Here's how the part is built. I have some questions about the finished solid (model axes, mm). Face numbers are marked on the shaded views. A direction names the side the tool comes from. Give positions to 0.01 mm unless a question says otherwise; leave off trailing zeros. Write each loop counter-clockwise with the first axis right and the second up, starting at its lowest first coordinate (ties: lowest second). Pieces come first, ordered by that corner, then holes. Notation, with made-up numbers: (-15.75, -35) - (-10.75, -35) arc R31 ccw to (-10.75, 4) - close; hole circle Ø7 at (84.25, -23). An arc over 180 degrees is marked (long way). Write each question's results on one line, items separated by ' | '. Start each with the question number.
Item 1: Suppose I cut it at A-A on y = 0. List the corners of the cut face in (x, z) for me (3 decimals).
Item 2: Suppose I cut it at C-C on y = -7. List the corners of the cut face in (x, z) for me, then the cut area to 3 significant figures.
Item 3: We'd pull the mould along Y, two halves only. Please class the marked faces 1, 2, 3 and 4: +Y half, -Y half, draft (parallel to the pull), parting line (faces both ways), or undercut.
Item 4: Suppose I cut it at D-D on x = -6.25. List the corners of the cut face in (y, z) for me, then the cut area to 3 significant figures.
Item 5: Which directions (+Z, -Z, +X, -X, +Y, -Y) give clear straight access to the entire face, cutting with the end or side of a thin tool? Please do the marked faces 5 and 6.
Item 6: Please list where these lines run through material, in increasing order: line 1 along Y through (x, z) = (0, 1.45) (3 decimals); line 2 along X through (y, z) = (0.25, 1.05); line 3 along Z through (x, y) = (8, -3.5).
Item 7: Will these pins go through, and if not, where does the flat tip stop? P1, Ø3.5, axis at x = 0, y = -7, coming from the +Z side; P2, Ø1.5, axis at y = 8, z = 0.5, coming from the -X side; P3, Ø1.5, axis at y = -4.5, z = 0.5, coming from the +X side.
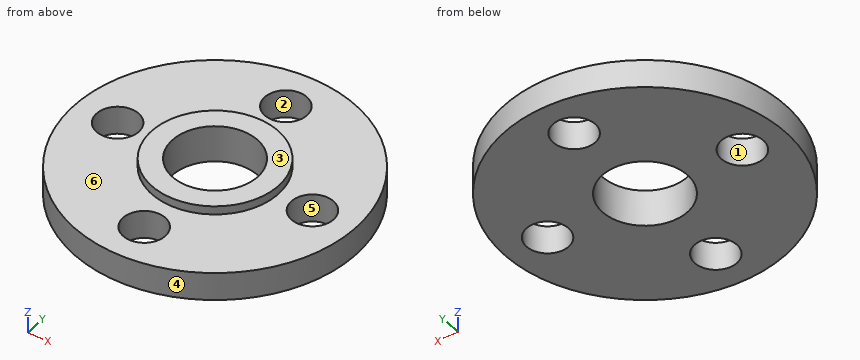
Autodesk Inventor part; units mm, degrees
ref_plane "YZ Plane" through (0, 0, 0) normal (1, 0, 0) x (0, 1, 0)
ref_plane "XZ Plane" through (0, 0, 0) normal (0, 1, 0) x (-1, 0, 0)
ref_plane "XY Plane" through (0, 0, 0) normal (0, 0, 1) x (1, 0, 0)
sketch "Sketch1" plane through (0, 0, 0) normal (0, 0, 1) x (1, 0, 0)
  circle A0 centre (0, 0) radius 10
  dimension "d0" = 20
extrude "Extrusion1" add sketch "Sketch1" along normal blind 2
sketch "Sketch2" plane through (0, 0, 2) normal (0, 0, 1) x (1, 0, 0)
  circle A0 centre (0, 0) radius 4.5
  dimension "d3" = 9
extrude "Extrusion2" add sketch "Sketch2" along normal blind 0.6
sketch "Sketch4" plane through (0, 0, 2.6) normal (0, 0, 1) x (1, 0, 0)
  circle A0 centre (0, 0) radius 3.025
  dimension "d9" = 6.05
extrude "Extrusion4" cut sketch "Sketch4" against normal through all
sketch "Sketch5" plane through (0, 0, 2) normal (0, 0, 1) x (1, 0, 0)
  line L0 (0, 0) -> (0, 7)
  circle A0 centre (0, 7) radius 1.5
  circle A1 centre (-7, 0) radius 1.5
  circle A2 centre (0, -7) radius 1.5
  circle A3 centre (7, 0) radius 1.5
  dimension "d12" = 7
  dimension "d13" = 3
  dimension "d16" = 360
extrude "Extrusion5" cut sketch "Sketch5" against normal through all
thread "Thread1"
thread "Thread2"
thread "Thread3"
thread "Thread4"
properties part number "servo_FT_SC_horn"
Checked values:
1) outline: (-10, 0) - (-8.5, 0) - (-8.5, 2) - (-10, 2) - close; (-5.5, 0) - (-3.025, 0) - (-3.025, 2.6) - (-4.5, 2.6) - (-4.5, 2) - (-5.5, 2) - close; (3.025, 0) - (5.5, 0) - (5.5, 2) - (4.5, 2) - (4.5, 2.6) - (3.025, 2.6) - close; (8.5, 0) - (10, 0) - (10, 2) - (8.5, 2) - close
2) outline: (-7.14, 0) - (-1.5, 0) - (-1.5, 2) - (-7.14, 2) - close; (1.5, 0) - (7.14, 0) - (7.14, 2) - (1.5, 2) - close | area: 22.6 mm^2
3) face 1: undercut | face 2: undercut | face 3: draft | face 4: parting line
4) outline: (-7.81, 0) - (-1.3, 0) - (-1.3, 2) - (-7.81, 2) - close; (1.3, 0) - (7.81, 0) - (7.81, 2) - (1.3, 2) - close | area: 26.0 mm^2
5) face 5: +Z, -Z | face 6: +Z
6) line 1: y = -10 to -8.5, -5.5 to -3.025, 3.025 to 5.5, 8.5 to 10 | line 2: x = -10 to -8.48, -5.52 to -3.01, 3.01 to 5.52, 8.48 to 10 | line 3: z = 0 to 2
7) P1: stops at z = 2 | P2: stops at x = -6.89 | P3: stops at x = 9.27
